Build history of the part. All positions in model axes, mm. Face numbers are marked on the shaded views. Round coordinates to 2 decimals unless told otherwise and drop trailing zeros. Order: outer loops, then holes, each group sorted by start corner. A loop starts at its lowest first (then second) coordinate and runs counter-clockwise, first axis right, second up. Notation, with made-up numbers: M 35.25,17.5 L 64.25,17.5 A17 cw 64.25,28.5 Z; hole C 51,-7.75 d8. An arc over 180 degrees is marked long. One line per item, written item: value. Start each with the question number.
Item 1: Pin check, flat tips, straight feed: pin 1 (0.8 mm diameter, centred on y = 21, z = -0.5, fed in from +X); pin 2 (1.8 mm diameter, centred on x = 57.5, y = 1, fed in from -Z); pin 3 (5 mm diameter, centred on x = -6.6, y = 39.5, fed in from -Z); pin 4 (0.8 mm diameter, centred on x = 44, z = -0.5, fed in from +Y). Stop position of each tip, or through.
Item 2: Probe L1, parallel to Y at x = 15.2, z = 0.85; L2, parallel to X at y = 39, z = 0.4; L3, parallel to Z at x = 50.5, y = 14.5. List the from-to ranges inside material, lowest first.
Item 3: Band-saw the part on C-C, the plane x = 15.2. Write the cut outline in (y, z), then the cut area to 3 significant figures.
Item 4: Band-saw the part on A-A, the plane x = 24. Write the cut outline in (y, z).
Item 5: Band-saw the part on B-B, the plane y = 9. Write the cut outline in (x, z), then the cut area to 3 significant figures.
Item 6: Two-plate mould, pull along Y, no slides. Class the marked faces 1 and 2: +Y half, -Y half, draft (parallel to the pull), parting line (faces both ways), or undercut.
Item 7: Band-saw the part on D-D, the plane y = 37.3. Give the number of separate pieces and of enclosed holes in the cut face, then the cut area to 3 significant figures.
```python
from build123d import *

# Parameters (mm, degrees)
SKETCH_2_R      = 1.5
SKETCH_2_R_2    = 1.6
EXTRUDE_1_DEPTH = 2
SKETCH_2_6_W    = 15
SKETCH_2_6_H    = 2
SKETCH_2_6_W_2  = 2
SKETCH_2_6_H_2  = 20.554974884
EXTRUDE_2_DEPTH = 1
FILLET_1_R      = 1


with BuildPart() as part:
    # 草图2 → 凸台-拉伸1 (new body)
    with BuildSketch(Plane.XY):
        with BuildLine():
            ThreePointArc((-10.601500464, -1), (-10.015714027, -2.414213562), (-8.601500464, -3))
            Line((-8.601500464, -3), (57.5, -3))
            ThreePointArc((57.5, -3), (61.5, 1), (57.5, 5))
            Line((57.5, 5), (55.5, 5))
            Line((55.5, 5), (55.5, 35.50095784))
            Line((55.5, 35.50095784), (58.590729836, 35.50095784))
            ThreePointArc((58.590729836, 35.50095784), (62.463713182, 38.50095784), (60.527221509, 43.00095784))
            Line((60.527221509, 43.00095784), (-8.601500464, 43.00095784))
            ThreePointArc((-8.601500464, 43.00095784), (-10.015714027, 42.415171403), (-10.601500464, 41.00095784))
            Line((-10.601500464, 41.00095784), (-10.601500464, -1))
        make_face()
        with Locations((-6.601500464, 1)):
            Circle(SKETCH_2_R, mode=Mode.SUBTRACT)
        with Locations((57.5, 1)):
            Circle(SKETCH_2_R, mode=Mode.SUBTRACT)
        with Locations((-6.601500464, 39.50095784)):
            Circle(SKETCH_2_R, mode=Mode.SUBTRACT)
        with Locations((15.2, 37.3)):
            Circle(SKETCH_2_R_2, mode=Mode.SUBTRACT)
        with Locations((23.5, 37.3)):
            Circle(SKETCH_2_R_2, mode=Mode.SUBTRACT)
        with Locations((58.590729836, 39.50095784)):
            Circle(SKETCH_2_R, mode=Mode.SUBTRACT)
    extrude(amount=EXTRUDE_1_DEPTH)

    # 草图2<6> → 凸台-拉伸2 (add)
    with BuildSketch(Plane.XY):
        with Locations((9.5, 40.50095784)):
            Rectangle(SKETCH_2_6_W, SKETCH_2_6_H)
        with Locations((-7.601500464, 22)):
            Rectangle(SKETCH_2_6_W_2, SKETCH_2_6_H_2)
        with Locations((43, 40.50095784)):
            Rectangle(SKETCH_2_6_W, SKETCH_2_6_H)
        with Locations((9.5, 0)):
            Rectangle(SKETCH_2_6_W, SKETCH_2_6_H)
        with Locations((43, 0)):
            Rectangle(SKETCH_2_6_W, SKETCH_2_6_H)
    extrude(amount=-EXTRUDE_2_DEPTH)

    # 圆角1
    # the kernel refuses this fillet: 1 mm, written as the material it takes off along each edge
    with BuildSketch(Plane(origin=(-8.601500464, -1, 2), x_dir=(-1, 0, 0), z_dir=(0, 1, 0))) as fillet_1_piece_1:
        with BuildLine():
            CenterArc((2 - FILLET_1_R, -FILLET_1_R), FILLET_1_R, 0, 90)
            Line((2 - FILLET_1_R, 0), (2, 0))
            Line((2, 0), (2, -FILLET_1_R))
        make_face()
    revolve(axis=Axis((-8.601500464, -1, 2), (0, 0, 1)), revolution_arc=90, mode=Mode.SUBTRACT)
    with BuildSketch(Plane(origin=(-8.601500464, -3, 2), x_dir=(0, 0, -1), z_dir=(1, 0, 0))) as fillet_1_piece_2:
        with BuildLine():
            CenterArc((FILLET_1_R, FILLET_1_R), FILLET_1_R, 180, 90)
            Line((0, FILLET_1_R), (0, 0))
            Line((0, 0), (FILLET_1_R, 0))
        make_face()
    extrude(amount=66.101500464, mode=Mode.SUBTRACT)
    with BuildSketch(Plane(origin=(57.5, 1, 2), x_dir=(0, -1, 0), z_dir=(-1, 0, 0))) as fillet_1_piece_3:
        with BuildLine():
            CenterArc((4 - FILLET_1_R, -FILLET_1_R), FILLET_1_R, 0, 90)
            Line((4, -FILLET_1_R), (4, 0))
            Line((4, 0), (4 - FILLET_1_R, 0))
        make_face()
    revolve(axis=Axis((57.5, 1, 2), (0, 0, 1)), revolution_arc=180, mode=Mode.SUBTRACT)
    with BuildSketch(Plane(origin=(57.5, 5, 2), x_dir=(0, -1, 0), z_dir=(-1, 0, 0))) as fillet_1_piece_4:
        with BuildLine():
            CenterArc((FILLET_1_R, -FILLET_1_R), FILLET_1_R, 90, 90)
            Line((0, -FILLET_1_R), (0, 0))
            Line((0, 0), (FILLET_1_R, 0))
        make_face()
    extrude(amount=2, mode=Mode.SUBTRACT)
    with BuildSketch(Plane(origin=(55.5, 5, 2), x_dir=(-1, 0, 0), z_dir=(0, 1, 0))) as fillet_1_piece_5:
        with BuildLine():
            CenterArc((FILLET_1_R, -FILLET_1_R), FILLET_1_R, 90, 90)
            Line((0, -FILLET_1_R), (0, 0))
            Line((0, 0), (FILLET_1_R, 0))
        make_face()
    extrude(amount=30.50095784, mode=Mode.SUBTRACT)
    with BuildSketch(Plane(origin=(55.5, 35.50095784, 2), x_dir=(0, 1, 0), z_dir=(1, 0, 0))) as fillet_1_piece_6:
        with BuildLine():
            CenterArc((FILLET_1_R, -FILLET_1_R), FILLET_1_R, 90, 90)
            Line((0, -FILLET_1_R), (0, 0))
            Line((0, 0), (FILLET_1_R, 0))
        make_face()
    extrude(amount=3.090729836, mode=Mode.SUBTRACT)
    with BuildSketch(Plane(origin=(58.590729836, 39.50095784, 2), x_dir=(0, -1, 0), z_dir=(-1, 0, 0))) as fillet_1_piece_7:
        with BuildLine():
            CenterArc((4 - FILLET_1_R, -FILLET_1_R), FILLET_1_R, 0, 90)
            Line((4, -FILLET_1_R), (4, 0))
            Line((4, 0), (4 - FILLET_1_R, 0))
        make_face()
    revolve(axis=Axis((58.590729836, 39.50095784, 2), (0, 0, 1)), revolution_arc=186.895375862, mode=Mode.SUBTRACT)
    with BuildSketch(Plane(origin=(63.027221509, 43.00095784, 2), x_dir=(0, -1, 0), z_dir=(-1, 0, 0))) as fillet_1_piece_8:
        with BuildLine():
            CenterArc((FILLET_1_R, -FILLET_1_R), FILLET_1_R, 90, 90)
            Line((0, -FILLET_1_R), (0, 0))
            Line((0, 0), (FILLET_1_R, 0))
        make_face()
    extrude(amount=71.628721973, mode=Mode.SUBTRACT)
    with BuildSketch(Plane(origin=(-8.601500464, 41.00095784, 2), x_dir=(0, 1, 0), z_dir=(1, 0, 0))) as fillet_1_piece_9:
        with BuildLine():
            CenterArc((2 - FILLET_1_R, -FILLET_1_R), FILLET_1_R, 0, 90)
            Line((2, -FILLET_1_R), (2, 0))
            Line((2, 0), (2 - FILLET_1_R, 0))
        make_face()
    revolve(axis=Axis((-8.601500464, 41.00095784, 2), (0, 0, 1)), revolution_arc=90, mode=Mode.SUBTRACT)
    with BuildSketch(Plane(origin=(-10.601500464, 41.00095784, 2), x_dir=(0, 0, -1), z_dir=(0, -1, 0))) as fillet_1_piece_10:
        with BuildLine():
            CenterArc((FILLET_1_R, FILLET_1_R), FILLET_1_R, 180, 90)
            Line((0, FILLET_1_R), (0, 0))
            Line((0, 0), (FILLET_1_R, 0))
        make_face()
    extrude(amount=42.00095784, mode=Mode.SUBTRACT)
    with BuildSketch(Plane(origin=(57.5, 5, 2), x_dir=(0, -1, 0), z_dir=(-1, 0, 0))) as fillet_1_piece_11a_section:
        with BuildLine():
            CenterArc((FILLET_1_R, -FILLET_1_R), FILLET_1_R, 90, 90)
            Line((0, -FILLET_1_R), (0, 0))
            Line((0, 0), (FILLET_1_R, 0))
        make_face()
    fillet_1_piece_11a = extrude(amount=4.5, mode=Mode.PRIVATE)
    fillet_1_piece_11a = split(fillet_1_piece_11a, bisect_by=Plane(origin=(55.5, 4.773604886, 1.773604886), z_dir=(-1, 0, 0)), keep=Keep.TOP, mode=Mode.PRIVATE)
    with BuildSketch(Plane(origin=(55.5, 2.5, 2), x_dir=(-1, 0, 0), z_dir=(0, 1, 0))) as fillet_1_piece_11b_section:
        with BuildLine():
            CenterArc((FILLET_1_R, -FILLET_1_R), FILLET_1_R, 90, 90)
            Line((0, -FILLET_1_R), (0, 0))
            Line((0, 0), (FILLET_1_R, 0))
        make_face()
    fillet_1_piece_11b = extrude(amount=33.00095784, mode=Mode.PRIVATE)
    fillet_1_piece_11b = split(fillet_1_piece_11b, bisect_by=Plane(origin=(55.273604886, 5, 1.773604886), z_dir=(0, -1, 0)), keep=Keep.TOP, mode=Mode.PRIVATE)
    fillet_1_piece_11 = fillet_1_piece_11a & fillet_1_piece_11b
    add(fillet_1_piece_11, mode=Mode.SUBTRACT)
    with BuildSketch(Plane(origin=(55.5, 5, 2), x_dir=(-1, 0, 0), z_dir=(0, 1, 0))) as fillet_1_piece_12a_section:
        with BuildLine():
            CenterArc((FILLET_1_R, -FILLET_1_R), FILLET_1_R, 90, 90)
            Line((0, -FILLET_1_R), (0, 0))
            Line((0, 0), (FILLET_1_R, 0))
        make_face()
    fillet_1_piece_12a = extrude(amount=33.00095784, mode=Mode.PRIVATE)
    fillet_1_piece_12a = split(fillet_1_piece_12a, bisect_by=Plane(origin=(55.273604886, 35.50095784, 1.773604886), z_dir=(0, 1, 0)), keep=Keep.TOP, mode=Mode.PRIVATE)
    with BuildSketch(Plane(origin=(53, 35.50095784, 2), x_dir=(0, 1, 0), z_dir=(1, 0, 0))) as fillet_1_piece_12b_section:
        with BuildLine():
            CenterArc((FILLET_1_R, -FILLET_1_R), FILLET_1_R, 90, 90)
            Line((0, -FILLET_1_R), (0, 0))
            Line((0, 0), (FILLET_1_R, 0))
        make_face()
    fillet_1_piece_12b = extrude(amount=5.590729836, mode=Mode.PRIVATE)
    fillet_1_piece_12b = split(fillet_1_piece_12b, bisect_by=Plane(origin=(55.5, 35.727352955, 1.773604886), z_dir=(-1, 0, 0)), keep=Keep.TOP, mode=Mode.PRIVATE)
    fillet_1_piece_12 = fillet_1_piece_12a & fillet_1_piece_12b
    add(fillet_1_piece_12, mode=Mode.SUBTRACT)


solid = part.part
```
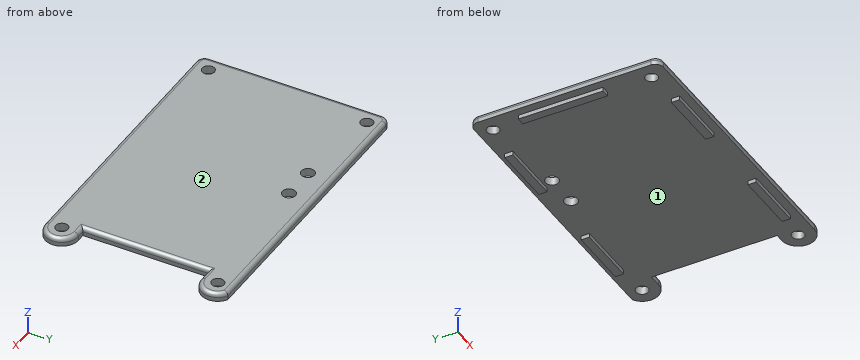
Output:
1. pin 1: stops at x = -6.6
1. pin 2: passes through
1. pin 3: stops at z = 0
1. pin 4: stops at y = 41.5
2. L1: y = -3 to 35.7, 38.9 to 43
2. L2: x = -10.6 to -8.02, -5.19 to 57.18, 60 to 62.56
2. L3: z = 0 to 2
3. outline: M -3,0 L -1,0 L -1,-1 L 1,-1 L 1,0 L 35.7,0 L 35.7,2 L -2,2 A1 ccw -3,1 Z; M 38.9,0 L 39.5,0 L 39.5,-1 L 41.5,-1 L 41.5,0 L 43,0 L 43,1 A1 ccw 42,2 L 38.9,2 Z
3. area: 89.2 mm²
4. outline: M -3,0 L 35.78,0 L 35.78,2 L -2,2 A1 ccw -3,1 Z; M 38.82,0 L 43,0 L 43,1 A1 ccw 42,2 L 38.82,2 Z
5. outline: M -10.6,0 L 55.5,0 L 55.5,1 A1 ccw 54.5,2 L -9.6,2 A1 ccw -10.6,1 Z
5. area: 132 mm²
6. face 1: undercut
6. face 2: draft
7. separate pieces: 3
7. enclosed holes: 0
7. area: 132 mm²
